```python
from build123d import *

# Parameters (mm, degrees)
SKETCH1_R           = 25
SKETCH1_R_2         = 20
BOSS_EXTRUDE1_DEPTH = 7.5
SKETCH4_R           = 6.5


with BuildPart() as part:
    # Sketch1 → Boss-Extrude1 (new, symmetric)
    with BuildSketch(Plane.XY):
        Circle(SKETCH1_R)
        Circle(SKETCH1_R_2, mode=Mode.SUBTRACT)
    extrude(amount=BOSS_EXTRUDE1_DEPTH, both=True)

    # Cut-Sweep2: sweep along a curve in space
    with BuildLine() as cut_sweep2_path:
        ThreePointArc((25, 0, 7.5), (17.67766953, 17.67766953, 7.5), (0, 25, 7.5))
        ThreePointArc((0, 25, 7.5), (-17.67766953, 17.67766953, 7.5), (-25, 0, 7.5))
        ThreePointArc((-25, 0, 7.5), (-17.67766953, -17.67766953, 7.5), (0, -25, 7.5))
        ThreePointArc((0, -25, 7.5), (17.67766953, -17.67766953, 7.5), (25, 0, 7.5))
    # Sketch4 → Cut-Sweep2 (sweep, cut)
    with BuildSketch(Plane(origin=(0, 0, 0), x_dir=(0, 0, -1), z_dir=(1, 0, 0))):
        with Locations((0, -30)):
            Circle(SKETCH4_R)
    sweep(path=cut_sweep2_path.line, mode=Mode.SUBTRACT)


solid = part.part
```
Geometry check sheet. Reference: the model listing, model coordinates, mm. Round coordinates to 2 decimals unless told otherwise and drop trailing zeros. Loops run counter-clockwise (first coordinate to the right, second up) from the corner with the lowest first, then second, coordinate; pieces in that order, holes last. Notation, with made-up numbers: M 70.5,24.5 L 88.5,24.5 A24 ccw 88.5,59.5 Z; hole C 46.5,65 d7. An arc over 180 degrees is marked long. Return JSON: item names as keys, results as strings. Group by question number.
(1) Go/stop test with flat-tipped pins: pin 1 (3 mm diameter, centred on x = -15.5, z = 2.5, fed in from -Y); pin 2 (2 mm diameter, centred on y = 12.5, z = 3.5, fed in from +X); pin 3 (6 mm diameter, centred on y = 15, z = 2, fed in from +X). Record where each tip stops, or that it passes through.
(2) Scan lines: line 1 along X through (y, z) = (-4, 6.75); line 2 along Y through (x, z) = (16.5, 3.25); line 3 along Y through (x, z) = (-10.5, 3.25). Record each from-to range of solid material in increasing order. Write a range as [from, to].
(3) Section check A-A, the plane z = -6. Enter the section's corners in (x, y).
(4) Section check C-C, the plane z = -0.75. Enter the section's corners in (x, y), and give its area (3 significant figures).
(5) Section check B-B, the plane z = 2. Enter the section's corners in (x, y).
(6) Mould release check, pull along X, two halves, no side actions. Record for faces 1 (the face through (-11, 17, -7.5)), 2 (the face through (23.846, 7.509, -5.803)), 3 (the face through (-4.336, -19.524, -0.105)): pulls with the +X half, pulls with the -X half, needs draft (parallel to the pull), parting line crosses it, or undercut.
Data:
{
 "1": {"pin 1": "y = -19.87", "pin 2": "x = 22.07", "pin 3": "x = 21.41"},
 "2": {"line 1": "[-24.68, -19.6], [19.6, 24.68]", "line 2": "[-17.94, -11.3], [11.3, 17.94]", "line 3": "[-21.99, -17.02], [17.02, 21.99]"},
 "3": {"outline": "C 0,0 d50; hole C 0,0 d40"},
 "4": {"outline": "C 0,0 d47.09; hole C 0,0 d40", "area": "485 mm²"},
 "5": {"outline": "C 0,0 d47.63; hole C 0,0 d40"},
 "6": {"face 1": "needs draft", "face 2": "parting line crosses it", "face 3": "undercut"}
}
